The model under review builds one solid part; all positions refer to its coordinate system, in mm. A direction names the side the tool comes from. Coordinates: 2 decimals unless noted, no trailing zeros. Write each loop counter-clockwise with the first axis right and the second up, starting at its lowest first coordinate (ties: lowest second). Pieces come first, ordered by that corner, then holes.
1) For line 1 (Y direction, x = -45.5, z = 51.5); line 2 (Y direction, x = -50, z = 32); line 3 (X direction, y = 15.5, z = 33), list the stretches that pass through material, from the lowest coordinate up.
2) Add section D-D, the plane x = 1.5. State the section outline as (y, z) points, then the cut area to 3 significant figures.
3) Add section B-B, the plane z = 36.5. State the section outline as (x, y) points, then the cut area to 3 significant figures.
4) Add section C-C, the plane x = 57.5. State the section outline as (y, z) points.
5) Mouldability with a two-part tool opening along Y and no side actions: class faces 4 (the flat face through (123.4, 7.96, 58.77)), 5 (the flat face through (-55, 38.593, 45)), 6 (the cylindrical face through (-38.959, 18.313, 22.306)) as released by +Y, released by -Y, zero draft, split by the parting line, or undercut.
6) For P1, Ø5.5, axis at y = 15, z = 57, coming from the +X side; P2, Ø6, axis at x = -49, y = 33, coming from the -Z side; P3, Ø5, axis at x = 70.5, z = 50, coming from the +Y side, all flat-tipped, find the tip position at first contact; note any pin that passes through.
7) Machinability: for faces 1 (the cylindrical face through (140.92, 19.03, 55.44)), 2 (the flat face through (-65, 28.443, 48)), 3 (the flat face through (123.33, 29.15, 58.77)), which of the approach directions +Z, -Z, +X, -X, +Y, -Y give a long, thin tool a straight path to every point of the face, cutting with its end or side? Answer none if there is none.
8) Add section A-A, the plane x = -67. State the section outline as (y, z) points.
from build123d import *

# Parameters (mm, degrees)
SKETCH1_R           = 2.73935274
BOSS_EXTRUDE1_DEPTH = 60
SKETCH16_R          = 2.1
SKETCH16_W          = 39.9
SKETCH16_H          = 19.7
CUT_EXTRUDE9_DEPTH  = 158.954623162
CUT_EXTRUDE11_DEPTH = 159.304157008
SKETCH19_W          = 123.088854382
SKETCH19_H          = 22
CUT_EXTRUDE12_DEPTH = 159.304157008
CUT_EXTRUDE14_DEPTH = 151.975703271
FILLET3_R           = 10
FILLET4_R           = 10
CUT_EXTRUDE15_DEPTH = 2.5


with BuildPart() as part:
    # Sketch1 → Boss-Extrude1 (new body)
    with BuildSketch(Plane.XY):
        with BuildLine():
            Line((-79.073756432, 38.59348199), (120.926243568, 38.59348199))
            ThreePointArc((120.926243568, 38.59348199), (140.926243568, 18.59348199), (120.926243568, -1.40651801))
            Line((120.926243568, -1.40651801), (-79.073756432, -1.40651801))
            ThreePointArc((-79.073756432, -1.40651801), (-99.073756432, 18.59348199), (-79.073756432, 38.59348199))
        make_face()
        with Locations((-79.073756432, 18.59348199)):
            Circle(SKETCH1_R, mode=Mode.SUBTRACT)
        with Locations((120.926243568, 18.59348199)):
            Circle(SKETCH1_R, mode=Mode.SUBTRACT)
    extrude(amount=BOSS_EXTRUDE1_DEPTH)

    # Sketch16 → Cut-Extrude9 (cut, through all)
    with BuildSketch(Plane.XY.offset(60)):
        with Locations((-93.68490205, 23.51848199)):
            Circle(SKETCH16_R)
        with Locations((-93.68490205, 13.66848199)):
            Circle(SKETCH16_R)
        with Locations((-44.262610814, 23.51848199)):
            Circle(SKETCH16_R)
        with Locations((-44.262610814, 13.66848199)):
            Circle(SKETCH16_R)
        with Locations((-68.973756432, 18.59348199)):
            Rectangle(SKETCH16_W, SKETCH16_H)
    extrude(amount=-CUT_EXTRUDE9_DEPTH, mode=Mode.SUBTRACT)

    # Sketch18 → Cut-Extrude11 (cut, through all)
    with BuildSketch(Plane(origin=(0, -1.40651801, 0), x_dir=(-1, 0, 0), z_dir=(0, -1, 0))):
        Polygon((-140.926243568, -55), (-140.926243568, 0), (-40.926243568, 0), align=None)
        Polygon((99.073756432, -55), (99.073756432, 0), (-0.926243568, 0), align=None)
    extrude(amount=-CUT_EXTRUDE11_DEPTH, mode=Mode.SUBTRACT)

    # Sketch19 → Cut-Extrude12 (cut, through all)
    with BuildSketch(Plane(origin=(0, -1.40651801, 0), x_dir=(-1, 0, 0), z_dir=(0, -1, 0))):
        with Locations((-19.381816377, -11)):
            Rectangle(SKETCH19_W, SKETCH19_H)
    extrude(amount=-CUT_EXTRUDE12_DEPTH, mode=Mode.SUBTRACT)

    # Sketch22 → Cut-Extrude14 (cut, through all)
    with BuildSketch(Plane(origin=(0, 0, 22), x_dir=(-1, 0, 0), z_dir=(0, 0, -1))):
        with BuildLine():
            Line((-80.926243568, 38.59348199), (39.073756432, 38.59348199))
            ThreePointArc((39.073756432, 38.59348199), (-20.926243568, 26.070752838), (-80.926243568, 38.59348199))
        make_face()
        with BuildLine():
            Line((-80.926243568, -1.40651801), (39.073756432, -1.40651801))
            ThreePointArc((39.073756432, -1.40651801), (-20.926243568, 11.116211141), (-80.926243568, -1.40651801))
        make_face()
    extrude(amount=-CUT_EXTRUDE14_DEPTH, mode=Mode.SUBTRACT)

    # Fillet3
    fillet3_edges = [part.edges().sort_by_distance(p)[0] for p in [
        (80.926243568, 18.59348199, 22),
    ]]
    fillet(fillet3_edges, radius=FILLET3_R)

    # Fillet4
    fillet4_edges = [part.edges().sort_by_distance(p)[0] for p in [
        (-39.073756432, 18.59348199, 22),
    ]]
    fillet(fillet4_edges, radius=FILLET4_R)

    # Sketch23 → Cut-Extrude15 (cut)
    with BuildSketch(Plane.XY.offset(60)):
        with BuildLine():
            Line((116.047109388, 31.94309545), (120.926243568, 26.438441465))
            Line((120.926243568, 26.438441465), (125.805377748, 31.94309545))
            ThreePointArc((125.805377748, 31.94309545), (128.926243568, 32.44988845), (130.047780865, 29.493742868))
            Line((130.047780865, 29.493742868), (127.720177765, 22.515961727))
            Line((127.720177765, 22.515961727), (134.926915045, 21.042834572))
            ThreePointArc((134.926915045, 21.042834572), (136.926243568, 18.59348199), (134.926915045, 16.144129408))
            Line((134.926915045, 16.144129408), (127.720177765, 14.671002252))
            Line((127.720177765, 14.671002252), (130.047780865, 7.693221111))
            ThreePointArc((130.047780865, 7.693221111), (128.926243568, 4.737075529), (125.805377748, 5.243868529))
            Line((125.805377748, 5.243868529), (120.926243568, 10.748522514))
            Line((120.926243568, 10.748522514), (116.047109388, 5.243868529))
            ThreePointArc((116.047109388, 5.243868529), (112.926243568, 4.737075529), (111.80470627, 7.693221111))
            Line((111.80470627, 7.693221111), (114.13230937, 14.671002252))
            Line((114.13230937, 14.671002252), (106.92557209, 16.144129408))
            ThreePointArc((106.92557209, 16.144129408), (104.926243568, 18.59348199), (106.92557209, 21.042834572))
            Line((106.92557209, 21.042834572), (114.13230937, 22.515961727))
            Line((114.13230937, 22.515961727), (111.80470627, 29.493742868))
            ThreePointArc((111.80470627, 29.493742868), (112.926243568, 32.44988845), (116.047109388, 31.94309545))
        make_face()
    extrude(amount=-CUT_EXTRUDE15_DEPTH, mode=Mode.SUBTRACT)


solid = part.part
Geometry results:
1. line 1: y = -1.41 to 11.97, 15.37 to 21.82, 25.22 to 38.59
1. line 2: y = -1.41 to 8.74, 28.44 to 38.59
1. line 3: x = -49.02 to -45.29, -43.24 to 100.93
2. outline: (9.85, 22) - (27.33, 22) - (27.33, 60) - (9.85, 60) - close
2. area: 664 mm2
3. outline: (-65.44, -1.41) - (-39.07, -1.41) arc R150 cw to (80.93, -1.41) - (107.29, -1.41) - (107.29, 38.59) - (80.93, 38.59) arc R150 cw to (-39.07, 38.59) - (-65.44, 38.59) - (-65.44, 28.44) - (-49.02, 28.44) - (-49.02, 8.74) - (-65.44, 8.74) - close; hole circle Ø4.2 at (-44.26, 13.67); hole circle Ø4.2 at (-44.26, 23.52)
3. area: 4,540 mm2
4. outline: (6.59, 22) - (30.6, 22) - (30.6, 60) - (6.59, 60) - close
5. face 4: undercut
5. face 5: released by +Y
5. face 6: zero draft
6. P1: stops at x = 140.91
6. P2: stops at z = 25.81
6. P3: stops at y = 35.4
7. face 1: +Z, -Z, +X
7. face 2: +Z, -Z
7. face 3: +Z
8. outline: (-1.41, 37.36) - (8.74, 37.36) - (8.74, 60) - (-1.41, 60) - close; (28.44, 37.36) - (38.59, 37.36) - (38.59, 60) - (28.44, 60) - close
